from build123d import *

# Parameters (mm, degrees)
F1_DEPTH = 25
F2_R     = 4.75
F3_DEPTH = 10
F4_R     = 7.6714476374
F5_DEPTH = 39.4


with BuildPart() as f1:
    # F0 (on Front) → F1 (new body)
    with BuildSketch(Plane.XZ):
        Polygon((-7.9714226845, 17.2469249544), (-18.92198649, 1.7200079281), (-10.9505638054, -15.5269170263), (7.9714226845, -17.2469249544), (18.92198649, -1.7200079281), (10.9505638054, 15.5269170263), align=None)
    extrude(amount=F1_DEPTH)

    # F2 (on face) → F3 (cut)
    with BuildSketch(Plane(origin=(-1.4895705605, 0, -16.3869209904), x_dir=(0.9958940258, 0, -0.0905267331), z_dir=(-0.0905267331, 0, -0.9958940258))):
        with Locations((0, 11.4799719304)):
            Circle(F2_R)
    extrude(amount=-F3_DEPTH, mode=Mode.SUBTRACT)

    # F4 (on face) → F5 (cut)
    with BuildSketch(Plane(origin=(14.9362751477, 0, 6.9034545491), x_dir=(0, 1, 0), z_dir=(0.9077328923, 0, 0.4195485623))):
        with Locations((-12.2148720548, 0)):
            Circle(F4_R)
    extrude(amount=-F5_DEPTH, mode=Mode.SUBTRACT)


solid = f1.part
Geometry: final body of the model. Coordinates: model frame, mm. Round coordinates to 2 decimals unless told otherwise and drop trailing zeros. Loops run counter-clockwise (first coordinate to the right, second up) from the corner with the lowest first, then second, coordinate; pieces in that order, holes last. Notation, with made-up numbers: M -6.75,-12.75 L 14.25,-12.75 A16 cw 14.25,-1.75 Z; hole C 36.5,27.25 d2. An arc over 180 degrees is marked long. One line per question, with ' | ' between items.
(1) Cut plane C-C on y = -23. Return the cut outline in (x, z).
Check result:
outline: M -18.92,1.72 L -10.95,-15.53 L 7.97,-17.25 L 18.92,-1.72 L 10.95,15.53 L -7.97,17.25 Z
(2) Contact query for flat-ended pins moving along their axis: P1, Ø8, axis at y = -20.5, z = -1.5, coming from the +X side; P2, Ø3, axis at y = -8.5, z = -9, coming from the +X side; P3, Ø1, axis at x = 3, y = -22, coming from the +Z side. Output: stop coordinate, or through.
Check result:
P1: stops at x = 18.92 | P2: stops at x = 14.85 | P3: stops at z = 16.3
(3) Material intervals for line 1 along Y through (x, z) = (0, -8.5); line 2 along Y through (x, z) = (-6.5, -7); line 3 along X through (y, z) = (-17, 15.5), sorted ascending. Write a range as from..to.
Check result:
line 1: y = -25..-16.17, -6.79..0 | line 2: y = -25..-18.97, -5.46..0 | line 3: x = -9.2..10.96
(4) Cut plane A-A on y = -16.75. Return the cut outline in (x, z).
Check result:
outline: M -18.92,1.72 L -17.53,-1.29 L 12.34,12.52 L 10.95,15.53 L -7.97,17.25 Z; M -12.34,-12.52 L -10.95,-15.53 L 7.97,-17.25 L 18.92,-1.72 L 17.53,1.29 Z
(5) Pull-direction query (X, two-part tool) for faces 1 (the cylindrical face through (-2.982, -13.214, 7.001)), 2 (the flat face through (13.37, -12.32, -9.59)), 3 (the flat face through (-13.37, -12.32, 9.59)); classes: +X half, -X half, draft (parallel to the pull), parting line (faces both ways), or undercut.
Check result:
face 1: undercut | face 2: +X half | face 3: -X half
(6) Cut plane B-B on y = -12.5. Return the cut outline in (x, z), plus the area to 3 significant figures.
Check result:
outline: M -18.92,1.72 L -18.15,0.06 L 11.72,13.86 L 10.95,15.53 L -7.97,17.25 Z; M -11.72,-13.86 L -10.95,-15.53 L -6.11,-15.97 L -5.66,-11.06 Z; M 3.13,-16.81 L 7.97,-17.25 L 18.92,-1.72 L 18.15,-0.06 L 3.55,-6.8 L 4.04,-6.85 Z | area: 363 mm2
